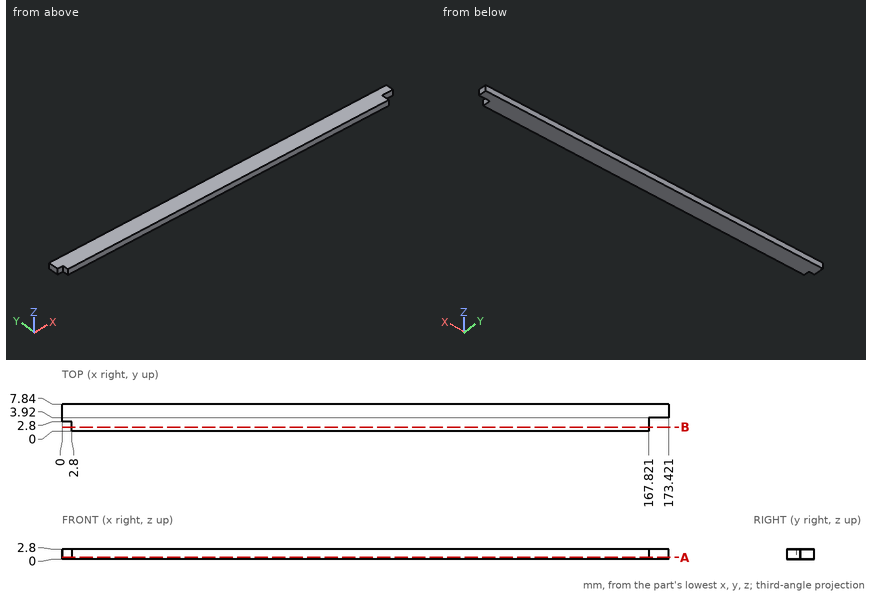
Can you work these out from the drawing? Everything is in mm from the part's minimum corner. Coordinates: 2 decimals unless noted, no trailing zeros. Write each loop counter-clockwise with the first axis right and the second up, starting at its lowest first coordinate (ties: lowest second). Pieces come first, ordered by that corner, then holes. Notation, with made-up numbers: (76, 36) -> (115, 36) arc R11 cw to (115, 54) -> close; hole circle Ø7 at (-28.75, 27.5). An arc over 180 degrees is marked (long way). Return JSON: item names as keys, results as strings.
(1) Imagine slicing it at A-A, the plane z = 0.55. Please give me the cut outline in (x, y), then the cut area to 3 significant figures.
Numbers:
{"outline": "(0, 2.8) -> (2.8, 2.8) -> (2.8, 0) -> (167.82, 0) -> (167.82, 3.92) -> (173.42, 3.92) -> (173.42, 7.84) -> (0, 7.84) -> close", "area": "1,330 mm2"}
(2) I'm going to push flat-ended pins straight in: pin 1 (1.4 mm diameter, centred on y = 2, z = 1, fed in from +X); pin 2 (1.4 mm diameter, centred on x = 1.5, z = 1, fed in from -Y); pin 3 (1 mm diameter, centred on y = 2, z = 0.5, fed in from -X). Where does each tip first touch, or does it pass through?
Numbers:
{"pin 1": "stops at x = 167.82", "pin 2": "stops at y = 2.8", "pin 3": "stops at x = 2.8"}
(3) I need wall thicknesses on L1, parallel to X at y = 2, z = 0.1. Which ranges of the line are inside material? Lowest first, please.
Numbers:
{"L1": "x = 2.8 to 167.82"}
(4) Imagine slicing it at B-B, the plane y = 1.25. Please give me the cut outline in (x, z), then the cut area to 3 significant figures.
Numbers:
{"outline": "(2.8, 0) -> (167.82, 0) -> (167.82, 2.8) -> (2.8, 2.8) -> close", "area": "462 mm2"}
